Read the model definition and answer for the solid it produces. Units are mm, in the model's axes. A direction names the side the tool comes from. Coordinates: 2 decimals unless noted, no trailing zeros. Write each loop counter-clockwise with the first axis right and the second up, starting at its lowest first coordinate (ties: lowest second). Pieces come first, ordered by that corner, then holes. Notation, with made-up numbers: (-5.5, -25.5) -> (-0.5, -25.5) arc R9 ccw to (-0.5, -14.5) -> close; hole circle Ø6 at (54, 84). An arc over 180 degrees is marked (long way). Answer as a JSON object with one key per item and string values. Group by question number.
(1) Which of the six approach directions +Z, -Z, +X, -X, +Y, -Y give full straight-line access (tool end or side, diameter ignored) to faces 4 (the face through (22.14, -21.6, 5.07)), 5 (the face through (0, -32.5, 5))?
(2) Find section A-A (y = -12.5). Give the vertices of the cut face in (x, z), then the cut area to 3 significant figures.
(3) Find section C-C (y = -1). Give the vertices of the cut face in (x, z).
(4) Find section D-D (x = 6.5). Give the vertices of the cut face in (y, z).
(5) Find section B-B (z = 5). Give the vertices of the cut face in (x, y).
(6) Flat-ended cylindrical pins translate along their axes: P1, Ø2, axis at y = -12.5, z = 5, coming from the +X side (1 decimal); P2, Ø3, axis at x = -2.5, z = 6.5, coming from the +Y side. Find the tip coordinate at first contact, or state that the pin passes through.
(7) For a pull along X with two mould halves and no side action, classify faces 1 (the face through (-23, 5, 5)), 2 (the face through (-25.54, -11.26, 4.84)), 3 (the face through (28, 0, 5)) as +X half, -X half, draft (parallel to the pull), parting line (faces both ways), or undercut.
(8) Straight lines are drawn through the part: L1, parallel to Y at x = -26.7, z = 5; L2, parallel to X at y = 20, z = 2; L3, parallel to Y at x = 25.15, z = 5. For each, find the intervals that lie inside material, in ascending order.
from build123d import *

# Parameters (mm, degrees)
EXTRUDE_1_DEPTH = 10
FILLET_1_R      = 3
M3X0_52_D       = 2.5


with BuildPart() as part:
    # Эскиз1 → Бобышка-Вытянуть1 (new body)
    with BuildSketch(Plane.XY):
        Polygon((28, 32.5), (23, 32.5), (23, -22.5), (-23, -22.5), (-23, 32.5), (-28, 32.5), (-28, -32.5), (28, -32.5), align=None)
    extrude(amount=EXTRUDE_1_DEPTH)

    # Скругление1
    fillet_1_edges = [part.edges().sort_by_distance(p)[0] for p in [
        (-23, 32.5, 5),
        (-23, -22.5, 5),
        (23, -22.5, 5),
        (23, 32.5, 5),
    ]]
    fillet(fillet_1_edges, radius=FILLET_1_R)

    # Отверстие обработанное метчиком M3x0.52 (through all)
    with Locations(Plane(origin=(28, 0, 0), x_dir=(0, 0, -1), z_dir=(1, 0, 0))):
        with Locations((-5, 22.5), (-5, -12.5)):
            Hole(M3X0_52_D / 2)


solid = part.part
Results below:
{
 "1": {"face 4": "+Z, -Z, +Y", "face 5": "+Z, -Z, +X, -X, -Y"},
 "2": {"outline": "(-28, 0) -> (-23, 0) -> (-23, 3.75) -> (-28, 3.75) -> close; (-28, 6.25) -> (-23, 6.25) -> (-23, 10) -> (-28, 10) -> close; (23, 0) -> (28, 0) -> (28, 3.75) -> (23, 3.75) -> close; (23, 6.25) -> (28, 6.25) -> (28, 10) -> (23, 10) -> close", "area": "75.0 mm2"},
 "3": {"outline": "(-28, 0) -> (-23, 0) -> (-23, 10) -> (-28, 10) -> close; (23, 0) -> (28, 0) -> (28, 10) -> (23, 10) -> close"},
 "4": {"outline": "(-32.5, 0) -> (-22.5, 0) -> (-22.5, 10) -> (-32.5, 10) -> close"},
 "5": {"outline": "(-28, -32.5) -> (28, -32.5) -> (28, -13.75) -> (23, -13.75) -> (23, -19.5) arc R3 cw to (20, -22.5) -> (-20, -22.5) arc R3 cw to (-23, -19.5) -> (-23, -13.75) -> (-28, -13.75) -> close; (-28, -11.25) -> (-23, -11.25) -> (-23, 21.25) -> (-28, 21.25) -> close; (-28, 23.75) -> (-23, 23.75) -> (-23, 29.5) arc R3 ccw to (-26, 32.5) -> (-28, 32.5) -> close; (23, -11.25) -> (28, -11.25) -> (28, 21.25) -> (23, 21.25) -> close; (23, 23.75) -> (28, 23.75) -> (28, 32.5) -> (26, 32.5) arc R3 ccw to (23, 29.5) -> close"},
 "6": {"P1": "passes through", "P2": "stops at y = -22.5"},
 "7": {"face 1": "undercut", "face 2": "draft", "face 3": "+X half"},
 "8": {"L1": "y = -32.5 to -13.75, -11.25 to 21.25, 23.75 to 32.5", "L2": "x = -28 to -23, 23 to 28", "L3": "y = -32.5 to -13.75, -11.25 to 21.25, 23.75 to 32.38"}
}
